from build123d import *

# Parameters (mm, degrees)
F0_W     = 550
F0_H     = 200
F0_R     = 9
F1_DEPTH = 30


with BuildPart() as f1:
    # F0 (on Top) → F1 (new body)
    with BuildSketch(Plane.XY):
        Rectangle(F0_W, F0_H)
        with Locations((-240, -41)):
            Circle(F0_R, mode=Mode.SUBTRACT)
        with Locations((240, -41)):
            Circle(F0_R, mode=Mode.SUBTRACT)
        with Locations((-240, 41)):
            Circle(F0_R, mode=Mode.SUBTRACT)
        with BuildLine():
            ThreePointArc((-42, 7), (-35, 0), (-42, -7))
            Line((-42, -7), (-152, -7))
            ThreePointArc((-152, -7), (-159, 0), (-152, 7))
            Line((-152, 7), (-42, 7))
        make_face(mode=Mode.SUBTRACT)
        with BuildLine():
            ThreePointArc((42, -7), (35, 0), (42, 7))
            Line((42, 7), (152, 7))
            ThreePointArc((152, 7), (159, 0), (152, -7))
            Line((152, -7), (42, -7))
        make_face(mode=Mode.SUBTRACT)
        with Locations((240, 41)):
            Circle(F0_R, mode=Mode.SUBTRACT)
    extrude(amount=-F1_DEPTH)


solid = f1.part
Here's how the part is built. I have some questions about the finished solid (model axes, mm). A direction names the side the tool comes from. Round coordinates to 2 decimals unless told otherwise and drop trailing zeros. Loops run counter-clockwise (first coordinate to the right, second up) from the corner with the lowest first, then second, coordinate; pieces in that order, holes last. Notation, with made-up numbers: (20.5, 18) - (55.5, 18) arc R16 ccw to (55.5, 35) - close; hole circle Ø9 at (35, 0.25). An arc over 180 degrees is marked (long way). One line per question, with ' | ' between items. Start each with the question number.
Q1. We'd pull the mould along Y, two halves only. Please class faces 3 (the flat face through (-4, -100, -15)), 4 (the flat face through (-98, 7, -15)), 5 (the cylindrical face through (35, 0, -15)), 6 (the flat face through (275, -1, -15)): +Y half, -Y half, draft (parallel to the pull), parting line (faces both ways), or undercut.
Q2. I want a section at A-A (z = -14.25). Write out the boundary of the cut face in (x, y).
Q3. I want a section at C-C (x = -240). Write out the boundary of the cut face in (y, z).
Q4. Please list where these lines run through material, in increasing order: line 1 (Y direction, x = 240, z = -15.5); line 2 (Y direction, x = -128.5, z = -7.5); line 3 (X direction, y = -2, z = -6). Write a range as [from, to].
Q5. I want a section at B-B (x = -123.5). Write out the boundary of the cut face in (y, z), then the cut area to 3 significant figures.
Q6. For faces 1 (the cylindrical face through (-159, 0, -15)), 2 (the flat face through (-4, 100, -15)), which set-ups out of +Z, -Z, +X, -X, +Y, -Y let a thin tool reach every point of the face, with its end or its side?
Response values:
1) face 3: -Y half | face 4: undercut | face 5: undercut | face 6: draft
2) outline: (-275, -100) - (275, -100) - (275, 100) - (-275, 100) - close; hole circle Ø18 at (-240, -41); hole circle Ø18 at (-240, 41); hole (-152, -7) - (-42, -7) arc R7 ccw to (-42, 7) - (-152, 7) arc R7 ccw to start; hole (42, -7) - (152, -7) arc R7 ccw to (152, 7) - (42, 7) arc R7 ccw to start; hole circle Ø18 at (240, -41); hole circle Ø18 at (240, 41)
3) outline: (-100, -30) - (-50, -30) - (-50, 0) - (-100, 0) - close; (-32, -30) - (32, -30) - (32, 0) - (-32, 0) - close; (50, -30) - (100, -30) - (100, 0) - (50, 0) - close
4) line 1: y = [-100, -50], [-32, 32], [50, 100] | line 2: y = [-100, -7], [7, 100] | line 3: x = [-275, -158.71], [-35.29, 35.29], [158.71, 275]
5) outline: (-100, -30) - (-7, -30) - (-7, 0) - (-100, 0) - close; (7, -30) - (100, -30) - (100, 0) - (7, 0) - close | area: 5,580 mm²
6) face 1: +Z, -Z | face 2: +Z, -Z, +X, -X, +Y
